Read the model definition and answer for the solid it produces. Units are mm, in the model's axes. Round coordinates to 2 decimals unless told otherwise and drop trailing zeros. Write each loop counter-clockwise with the first axis right and the second up, starting at its lowest first coordinate (ties: lowest second). Pieces come first, ordered by that corner, then holes. Notation, with made-up numbers: (88, -6) - (100, -6) arc R26 cw to (100, 16) - close; hole circle Ø11 at (39, 3). An arc over 180 degrees is marked (long way). Answer as CSV lines item,"result". Start each with the question number.
1) Each of these flat-tipped pins is pushed along its axis until it touches: pin 1 (2 mm diameter, centred on x = -14.85, y = -19.09, fed in from -Z); pin 2 (2 mm diameter, centred on x = 28, z = 4.5, fed in from +Y); pin 3 (1 mm diameter, centred on x = -6.5, z = 3.5, fed in from +Y); pin 4 (3 mm diameter, centred on y = -5.5, z = 7.5, fed in from -X). Where does it stop, or does it pass through?
2) Find section D-D on x = 34. Determine the outline of the cut face in (y, z), then the cut area to 3 significant figures.
3) Consider line 1 along Y through (x, z) = (-14.5, 2); line 2 along Y through (x, z) = (29.5, 7.5); line 3 along X through (y, z) = (-9, 4.5). Determine where each line is inside the solid, lowest interval first.
4) Find section B-B on z = 8. State how many separate pieces and enclosed holes the cut face has, then the cut area to 3 significant figures.
5) Find section A-A on y = 8. Determine the outline of the cut face in (x, z).
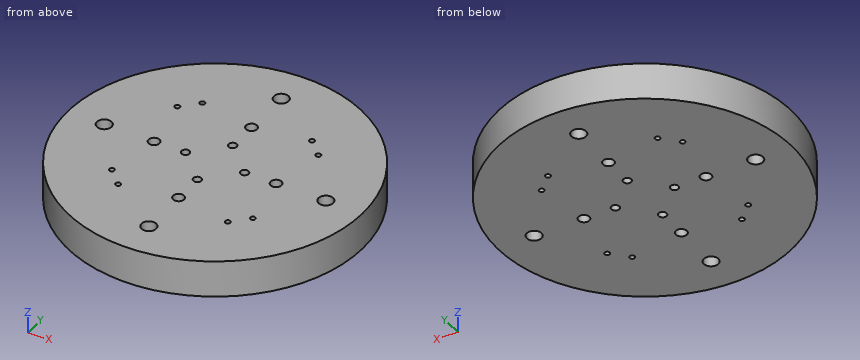
from build123d import *

# Parameters (mm, degrees)
SKETCH1_R                      = 40
BOSS_EXTRUDE1_DEPTH            = 10
F_4_0_4_DIAMETER_HOLE1_D       = 4
F_4_0_4_DIAMETER_HOLE1_DEPTH   = 10
F_4_0_4_DIAMETER_HOLE1_TIP     = 1.201721238
F_2_2_2_2_DIAMETER_HOLE1_D     = 2.2
F_2_2_2_2_DIAMETER_HOLE1_DEPTH = 10
F_2_2_2_2_DIAMETER_HOLE1_TIP   = 0.660946681
F_3_0_3_DIAMETER_HOLE4_D       = 3
F_3_0_3_DIAMETER_HOLE4_DEPTH   = 10
F_3_0_3_DIAMETER_HOLE4_TIP     = 0.901290929
F_1_4_1_4_DIAMETER_HOLE1_D     = 1.4
CIRPATTERN1_COUNT              = 4


with BuildPart() as part:
    # Sketch1 → Boss-Extrude1 (new body)
    with BuildSketch(Plane.XY):
        Circle(SKETCH1_R)
    extrude(amount=BOSS_EXTRUDE1_DEPTH)

    # Ø4.0 (4) Diameter Hole1
    with Locations(Plane.XY.offset(10)):
        with Locations((0, 30), (30, 0), (-30, 0), (0, -30)):
            Hole(F_4_0_4_DIAMETER_HOLE1_D / 2, depth=F_4_0_4_DIAMETER_HOLE1_DEPTH)
            with Locations((0, 0, -(F_4_0_4_DIAMETER_HOLE1_DEPTH + F_4_0_4_DIAMETER_HOLE1_TIP / 2))):  # 118° drill point
                Cone(0, F_4_0_4_DIAMETER_HOLE1_D / 2, F_4_0_4_DIAMETER_HOLE1_TIP, mode=Mode.SUBTRACT)

    # Ø2.2 (2.2) Diameter Hole1
    with Locations(Plane.XY.offset(10)):
        with Locations((0, 8), (0, -8), (-8, 0), (8, 0)):
            Hole(F_2_2_2_2_DIAMETER_HOLE1_D / 2, depth=F_2_2_2_2_DIAMETER_HOLE1_DEPTH)
            with Locations((0, 0, -(F_2_2_2_2_DIAMETER_HOLE1_DEPTH + F_2_2_2_2_DIAMETER_HOLE1_TIP / 2))):  # 118° drill point
                Cone(0, F_2_2_2_2_DIAMETER_HOLE1_D / 2, F_2_2_2_2_DIAMETER_HOLE1_TIP, mode=Mode.SUBTRACT)

    # Ø3.0 (3) Diameter Hole4
    with Locations(Plane.XY.offset(10)):
        with Locations((0, -16.52447999), (16.52447999, 0), (0, 16.52447999), (-16.52447999, 0)):
            Hole(F_3_0_3_DIAMETER_HOLE4_D / 2, depth=F_3_0_3_DIAMETER_HOLE4_DEPTH)
            with Locations((0, 0, -(F_3_0_3_DIAMETER_HOLE4_DEPTH + F_3_0_3_DIAMETER_HOLE4_TIP / 2))):  # 118° drill point
                Cone(0, F_3_0_3_DIAMETER_HOLE4_D / 2, F_3_0_3_DIAMETER_HOLE4_TIP, mode=Mode.SUBTRACT)

    # Ø1.4 (1.4) Diameter Hole1 (through all)
    with Locations(Plane.XY.offset(10)):
        with Locations((-14.849242405, -19.091883092), (-19.091883092, -14.849242405)):
            f_1_4_1_4_diameter_hole1 = Hole(F_1_4_1_4_DIAMETER_HOLE1_D / 2)

    # CirPattern1: Ø1.4 (1.4) Diameter Hole1 ×4 about axis
    cirpattern1_axis = Axis((0, 0, 0), (0, 0, 1))
    for i in range(1, CIRPATTERN1_COUNT):
        add(f_1_4_1_4_diameter_hole1.rotate(cirpattern1_axis, i * 360 / CIRPATTERN1_COUNT), mode=Mode.SUBTRACT)


solid = part.part
Check values:
1,pin 1,"stops at z = 0"
1,pin 2,"stops at y = 29.51"
1,pin 3,"stops at y = 39.55"
1,pin 4,"stops at x = -39.8"
2,outline,"(-21.07, 0) - (21.07, 0) - (21.07, 10) - (-21.07, 10) - close"
2,area,"421 mm^2"
3,line 1,"y = -37.28 to -19.7, -18.49 to 18.49, 19.7 to 37.28"
3,line 2,"y = -27.01 to -1.94, 1.94 to 27.01"
3,line 3,"x = -38.97 to -0.46, 0.46 to 38.97"
4,separate pieces,"1"
4,enclosed holes,"20"
4,area,"4,920 mm^2"
5,outline,"(-39.19, 0) - (-1.1, 0) - (-1.1, 10) - (-39.19, 10) - close; (1.1, 0) - (39.19, 0) - (39.19, 10) - (1.1, 10) - close"
